Can you work these out from the model? Positions are in its coordinate system, mm. A direction names the side the tool comes from. Round coordinates to 2 decimals unless told otherwise and drop trailing zeros. Order: outer loops, then holes, each group sorted by start corner. A loop starts at its lowest first (then second) coordinate and runs counter-clockwise, first axis right, second up. Notation, with made-up numbers: (-4, 68.5) -> (21, 68.5) arc R20 ccw to (21, 94.5) -> close; hole circle Ø8 at (44, 64). An arc over 180 degrees is marked (long way). Use a Markdown table: item, result. Add a question column.
Q1. For faces 1 (the face through (-13.951, 3.214, -5.423)), 2 (the face through (-12.92, 7.85, -45.55)), 3 (the face through (-5, 12, -28.5)), which set-ups out of +Z, -Z, +X, -X, +Y, -Y let a thin tool reach every point of the face, with its end or its side?
Q2. I'm going to push flat-ended pins straight in: pin 1 Ø10 at (x, y) = (-51.5, 14.5) entering from +Z; pin 2 Ø10 at (y, z) = (7, -50.5) entering from -X; pin 3 Ø24 at (x, z) = (-40, -30) entering from -Y; pin 4 Ø12 at (y, z) = (13.5, -10.5) entering from -X. Where does each tip first touch, or does it pass through?
Q3. We'd pull the mould along Z, two halves only. Please class faces 4 (the face through (-25, 12, 0)), 5 (the face through (-20, 24, -37)), 6 (the face through (-8, 9, -31.5)): +Z half, -Z half, draft (parallel to the pull), parting line (faces both ways), or undercut.
Q4. If we section it at B-B on z = -42.5: List the corners of the cut face in (x, y) for me.
Q5. If we section it at D-D on x = -28: List the corners of the cut face in (y, z) for me.
Q6. If we section it at A-A on y = 12: List the corners of the cut face in (x, z) for me, plus the area to 3 significant figures.
Q7. If we section it at C-C on x = -12: List the corners of the cut face in (y, z) for me, plus the area to 3 significant figures.
Q8. I need wall thicknesses on line 1 along Y through (x, z) = (-12, -8); line 2 along X through (y, z) = (14.25, -34.5); line 3 along X through (y, z) = (10, -42). Which ranges of each line are inside material? Lowest first, please. Write a range as [from, to].
```python
from build123d import *

# Parameters (mm, degrees)
P_IDAT_VYSUNUT_M1_DEPTH  = 24
ODEBRAT_VYSUNUT_M1_REACH = 62
SKICA2_R                 = 5.5
SKICA3_R                 = 9
ODEBRAT_VYSUNUT_M2_DEPTH = 11
M10_Z_VIT1_D             = 8.5
M10_Z_VIT1_DEPTH         = 28.5


with BuildPart() as part:
    # Skica1 → Přidat vysunutím1 (new body)
    with BuildSketch(Plane(origin=(0, 0, 0), x_dir=(1, 0, 0), z_dir=(0, 1, 0))):
        with BuildLine():
            Line((0, 0), (0, 28.5))
            Line((0, 28.5), (-20.056329325, 28.5))
            ThreePointArc((-20.056329325, 28.5), (-60, 30), (-20.056329325, 31.5))
            Line((-20.056329325, 31.5), (0, 31.5))
            Line((0, 31.5), (0, 60))
            Line((0, 60), (-40, 60))
            ThreePointArc((-40, 60), (-70, 30), (-40, 0))
            Line((-40, 0), (0, 0))
        make_face()
    extrude(amount=P_IDAT_VYSUNUT_M1_DEPTH)

    # Skica2 → Odebrat vysunutím1 (cut, up to next)
    with BuildSketch(Plane.XY, mode=Mode.PRIVATE) as odebrat_vysunut_m1_sk1:
        with Locations((-12, 12)):
            Circle(SKICA2_R)
    odebrat_vysunut_m1_tool1 = extrude(odebrat_vysunut_m1_sk1.sketch, amount=-ODEBRAT_VYSUNUT_M1_REACH, mode=Mode.PRIVATE) & part.part
    add(odebrat_vysunut_m1_tool1.solids().sort_by_distance((-12, 12, 0))[0], mode=Mode.SUBTRACT)

    # Skica3 → Odebrat vysunutím2 (cut)
    with BuildSketch(Plane.XY):
        with Locations((-12, 12)):
            Circle(SKICA3_R)
    extrude(amount=-ODEBRAT_VYSUNUT_M2_DEPTH, mode=Mode.SUBTRACT)

    # M10 závit1
    with Locations(Plane(origin=(0, 0, -60), x_dir=(-1, 0, 0), z_dir=(0, 0, -1))):
        with Locations((12, 12)):
            Hole(M10_Z_VIT1_D / 2, depth=M10_Z_VIT1_DEPTH)


solid = part.part
```
Answer below:
| question | item | result |
|---|---|---|
| 1 | face 1 | +Z |
| 1 | face 2 | +Z, -Z |
| 1 | face 3 | +X, +Y, -Y |
| 2 | pin 1 | z = -0.71 |
| 2 | pin 2 | x = -65.69 |
| 2 | pin 3 | through |
| 2 | pin 4 | x = -66.79 |
| 3 | face 4 | +Z half |
| 3 | face 5 | draft |
| 3 | face 6 | undercut |
| 4 | outline | (-67.27, 0) -> (-55.61, 0) -> (-55.61, 24) -> (-67.27, 24) -> close; (-24.39, 0) -> (0, 0) -> (0, 24) -> (-24.39, 24) -> close; hole circle Ø8.5 at (-12, 12) |
| 5 | outline | (0, -60) -> (24, -60) -> (24, -46) -> (0, -46) -> close; (0, -14) -> (24, -14) -> (24, 0) -> (0, 0) -> close |
| 6 | outline | (-40, -60) -> (-16.25, -60) -> (-16.25, -31.5) -> (-20.06, -31.5) arc R20 cw (long way) to (-20.06, -28.5) -> (-17.5, -28.5) -> (-17.5, -11) -> (-21, -11) -> (-21, 0) -> (-40, 0) arc R30 ccw to start; (-7.75, -60) -> (0, -60) -> (0, -31.5) -> (-7.75, -31.5) -> close; (-6.5, -28.5) -> (0, -28.5) -> (0, 0) -> (-3, 0) -> (-3, -11) -> (-6.5, -11) -> close |
| 6 | area | 1,860 mm² |
| 7 | outline | (0, -60) -> (7.75, -60) -> (7.75, -31.5) -> (0, -31.5) -> close; (0, -28.5) -> (6.5, -28.5) -> (6.5, -11) -> (3, -11) -> (3, 0) -> (0, 0) -> close; (16.25, -60) -> (24, -60) -> (24, -31.5) -> (16.25, -31.5) -> close; (17.5, -28.5) -> (24, -28.5) -> (24, 0) -> (21, 0) -> (21, -11) -> (17.5, -11) -> close |
| 7 | area | 735 mm² |
| 8 | line 1 | [0, 3], [21, 24] |
| 8 | line 2 | [-69.66, -59.49], [-20.51, -15.61], [-8.39, 0] |
| 8 | line 3 | [-67.5, -56], [-24, -15.75], [-8.25, 0] |
